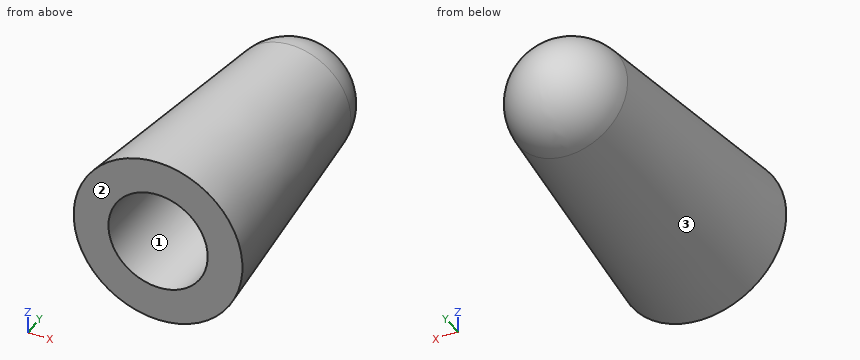
from build123d import *


with BuildPart() as part:
    # Esquisse1 → Révolution1 (revolve)
    with BuildSketch(Plane.XY, mode=Mode.PRIVATE) as r_volution1_sk:
        with BuildLine():
            Line((-2.5, 0), (-4.25, 0))
            Line((-4.25, 0), (-2.984258228, 12.306924789))
            ThreePointArc((-2.984258228, 12.306924789), (-2.009878806, 14.227192669), (0, 15))
            Line((0, 15), (0, 14))
            ThreePointArc((0, 14), (-1.414213562, 13.414213562), (-2, 12))
            Line((-2, 12), (-2, 6))
            Line((-2, 6), (-2.5, 6))
            Line((-2.5, 6), (-2.5, 0))
        make_face()
    revolve(r_volution1_sk.sketch.rotate(Axis((0, 0, 0), (0, 1, 0)), 270), axis=Axis((0, 0, 0), (0, 1, 0)))  # turned: the seam where the file's is


solid = part.part
Here's how the part is built. I have some questions about the finished solid (model axes, mm). Face numbers are marked on the shaded views. Coordinates: 2 decimals unless noted, no trailing zeros. Write each loop counter-clockwise with the first axis right and the second up, starting at its lowest first coordinate (ties: lowest second). Pieces come first, ordered by that corner, then holes.
1) If we section it at C-C (y = 5.25): List the corners of the cut face in (x, z) for me, plus the area to 3 significant figures.
Filled in:
outline: circle Ø7.42 at (0, 0); hole circle Ø5 at (0, 0)
area: 23.6 mm2
2) If we section it at A-A (x = 0): List the corners of the cut face in (y, z) for me, plus the area to 3 significant figures.
Filled in:
outline: (0, -4.25) - (12.31, -2.98) arc R3 ccw to (12.31, 2.98) - (0, 4.25) - (0, 2.5) - (6, 2.5) - (6, 2) - (12, 2) arc R2 cw to (12, -2) - (6, -2) - (6, -2.5) - (0, -2.5) - close
area: 41.0 mm2
3) If I drill on line 1 (Z direction, x = 1.75, y = 2.25); line 2 (Z direction, x = 1.75, y = 9.25); line 3 (X direction, y = 8.05, z = 0), over which ranges is the centre line in solid material (lowest first)?
Filled in:
line 1: z = -3.62 to -1.79, 1.79 to 3.62
line 2: z = -2.8 to -0.97, 0.97 to 2.8
line 3: x = -3.42 to -2, 2 to 3.42
4) I'm going to push flat-ended pins straight in: pin 1 (2.5 mm diameter, centred on x = 0, z = 0.5, fed in from -Y); pin 2 (3 mm diameter, centred on y = 5.5, z = 1.5, fed in from +X); pin 3 (1.5 mm diameter, centred on y = 9.5, z = 1.5, fed in from +X). Where does each tip first touch, or does it pass through?
Filled in:
pin 1: stops at y = 12.97
pin 2: stops at x = 3.77
pin 3: stops at x = 3.2
5) If we section it at B-B (y = 7.75): List the corners of the cut face in (x, z) for me.
Filled in:
outline: circle Ø6.91 at (0, 0); hole circle Ø4 at (0, 0)
6) Thinking about a two-plate mould opening in X: for the marked faces 1, 2 and 3, which applies, +X half, -X half, draft (parallel to the pull), parting line (faces both ways), or undercut?
Filled in:
face 1: undercut
face 2: draft
face 3: parting line
